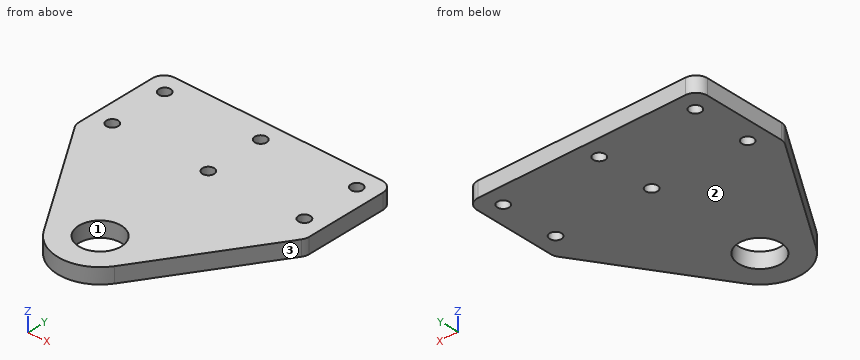
from build123d import *

# Parameters (mm, degrees)
SKETCH_1_R          = 5.5
EXTRUDE_1_DEPTH     = 4
FILLET_1_R          = 3
SKETCH_3_R          = 1.525
CUT_EXTRUDE_2_DEPTH = 10


with BuildPart() as part:
    # 草图1 → 凸台-拉伸1 (new body)
    with BuildSketch(Plane.XY):
        with BuildLine():
            Line((-9.225454443, -5.990908973), (-30, 26))
            Line((-30, 26), (-30, 51))
            Line((-30, 51), (30, 51))
            Line((30, 51), (30, 26))
            Line((30, 26), (9.225454443, -5.990908973))
            ThreePointArc((9.225454443, -5.990908973), (0, -11), (-9.225454443, -5.990908973))
        make_face()
        Circle(SKETCH_1_R, mode=Mode.SUBTRACT)
    extrude(amount=EXTRUDE_1_DEPTH)

    # 圆角1
    fillet_1_edges = [part.edges().sort_by_distance(p)[0] for p in [
        (-30, 26, 2),
        (-30, 51, 2),
        (30, 51, 2),
        (30, 26, 2),
    ]]
    fillet(fillet_1_edges, radius=FILLET_1_R)

    # 草图3 → 切除-拉伸2 (cut)
    with BuildSketch(Plane(origin=(0, 0, 0), x_dir=(-1, 0, 0), z_dir=(0, 0, -1))):
        with Locations((25, 31)):
            Circle(SKETCH_3_R)
        with Locations((25, 46)):
            Circle(SKETCH_3_R)
        with Locations((0, 31)):
            Circle(SKETCH_3_R)
        with Locations((0, 46)):
            Circle(SKETCH_3_R)
        with Locations((-25, 31)):
            Circle(SKETCH_3_R)
        with Locations((-25, 46)):
            Circle(SKETCH_3_R)
    extrude(amount=-CUT_EXTRUDE_2_DEPTH, mode=Mode.SUBTRACT)


solid = part.part
Could you check a few things on this model? Use its own coordinates, in mm. Face numbers are marked on the shaded views. Round coordinates to 2 decimals unless told otherwise and drop trailing zeros. Write each loop counter-clockwise with the first axis right and the second up, starting at its lowest first coordinate (ties: lowest second). Pieces come first, ordered by that corner, then holes. Notation, with made-up numbers: (12, 11.25) -> (26, 11.25) arc R23 ccw to (26, 45.25) -> close; hole circle Ø2 at (-4.5, 76). An arc over 180 degrees is marked (long way). Use a Markdown table: item, result.
1. If we section it at A-A (x = 0): List the corners of the cut face in (y, z) for me (3 decimals), then the cut area to 3 significant figures.
Answer key:
| item | result |
|---|---|
| outline | (-11, 0) -> (-5.5, 0) -> (-5.5, 4) -> (-11, 4) -> close; (5.5, 0) -> (29.475, 0) -> (29.475, 4) -> (5.5, 4) -> close; (32.525, 0) -> (44.475, 0) -> (44.475, 4) -> (32.525, 4) -> close; (47.525, 0) -> (51, 0) -> (51, 4) -> (47.525, 4) -> close |
| area | 180 mm^2 |
2. For pin 1 Ø2 at (y, z) = (15.5, 3.5) entering from +X; pin 2 Ø1 at (x, z) = (6.5, 1) entering from -Y; pin 3 Ø1 at (x, z) = (10, 1) entering from -Y, each with a flat end and sliding along its axis, tell me the tip position at first contact or that it passes through.
Answer key:
| item | result |
|---|---|
| pin 1 | stops at x = 23.83 |
| pin 2 | stops at y = -9.22 |
| pin 3 | stops at y = -5.57 |
3. We'd pull the mould along Y, two halves only. Please class the marked faces 1, 2 and 3: +Y half, -Y half, draft (parallel to the pull), parting line (faces both ways), or undercut.
Answer key:
| item | result |
|---|---|
| face 1 | undercut |
| face 2 | draft |
| face 3 | -Y half |
4. If we section it at C-C (y = 31): List the corners of the cut face in (x, z) for me (3 decimals), then the cut area to 3 significant figures.
Answer key:
| item | result |
|---|---|
| outline | (-30, 0) -> (-26.525, 0) -> (-26.525, 4) -> (-30, 4) -> close; (-23.475, 0) -> (-1.525, 0) -> (-1.525, 4) -> (-23.475, 4) -> close; (1.525, 0) -> (23.475, 0) -> (23.475, 4) -> (1.525, 4) -> close; (26.525, 0) -> (30, 0) -> (30, 4) -> (26.525, 4) -> close |
| area | 203 mm^2 |
5. If we section it at D-D (x = 25): List the corners of the cut face in (y, z) for me (3 decimals), then the cut area to 3 significant figures.
Answer key:
| item | result |
|---|---|
| outline | (18.3, 0) -> (29.475, 0) -> (29.475, 4) -> (18.3, 4) -> close; (32.525, 0) -> (44.475, 0) -> (44.475, 4) -> (32.525, 4) -> close; (47.525, 0) -> (51, 0) -> (51, 4) -> (47.525, 4) -> close |
| area | 106 mm^2 |
6. If we section it at B-B (z = 1.1): List the corners of the cut face in (x, y) for me (3 decimals).
Answer key:
| item | result |
|---|---|
| outline | (-30, 26.889) arc R3 ccw to (-29.516, 25.255) -> (-9.225, -5.991) arc R11 ccw to (9.225, -5.991) -> (29.516, 25.255) arc R3 ccw to (30, 26.889) -> (30, 48) arc R3 ccw to (27, 51) -> (-27, 51) arc R3 ccw to (-30, 48) -> close; hole circle Ø3.05 at (-25, 31); hole circle Ø3.05 at (-25, 46); hole circle Ø11 at (0, 0); hole circle Ø3.05 at (0, 31); hole circle Ø3.05 at (0, 46); hole circle Ø3.05 at (25, 31); hole circle Ø3.05 at (25, 46) |
7. Please list where these lines run through material, in increasing order: probe 1 along Y at (x, z) = (0, 1.6) (3 decimals); probe 2 along Y at (x, z) = (-25, 2.25) (3 decimals); probe 3 along Y at (x, z) = (-25.5, 1.7).
Answer key:
| item | result |
|---|---|
| probe 1 | y = -11 to -5.5, 5.5 to 29.475, 32.525 to 44.475, 47.525 to 51 |
| probe 2 | y = 18.3 to 29.475, 32.525 to 44.475, 47.525 to 51 |
| probe 3 | y = 19.07 to 29.56, 32.44 to 44.56, 47.44 to 51 |
